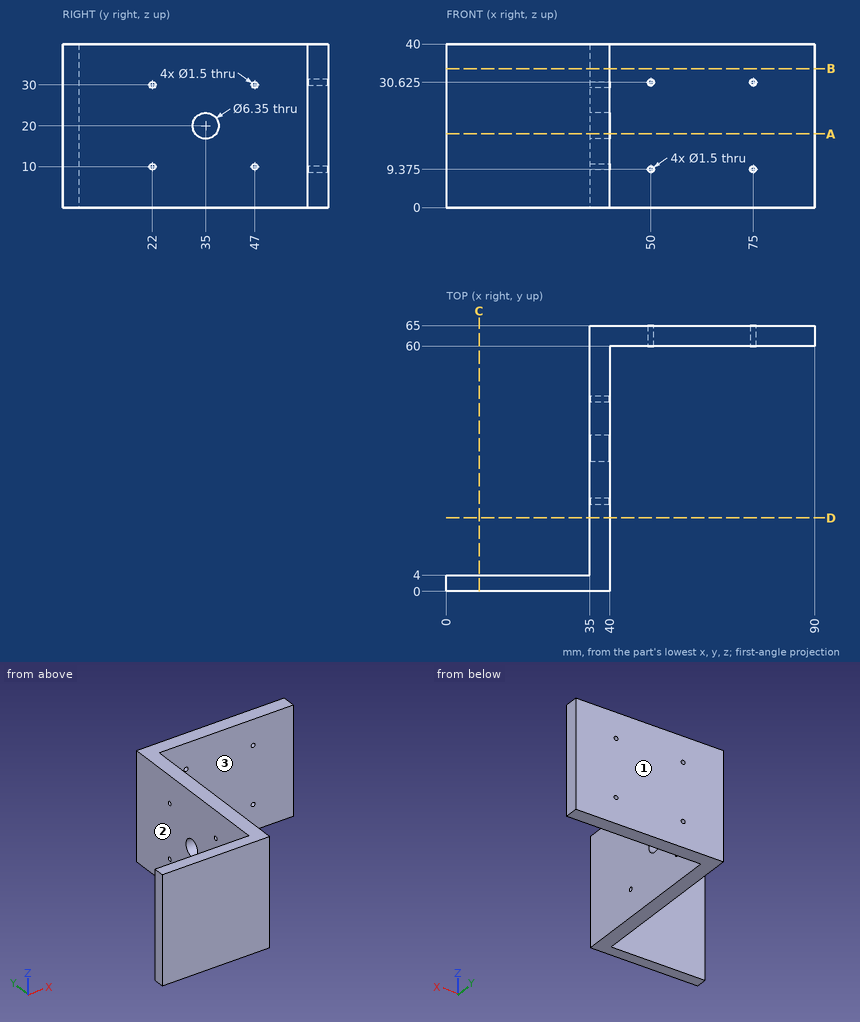
Geometry check sheet. Reference: drawing and pictorial views, mm from the part's lowest x, y, z. A direction names the side the tool comes from. Round coordinates to 2 decimals unless told otherwise and drop trailing zeros. Write each loop counter-clockwise with the first axis right and the second up, starting at its lowest first coordinate (ties: lowest second). Pieces come first, ordered by that corner, then holes.
Item 1: Section check A-A (z = 18). Record the boundary of the cut face in (x, y), plus the area to 3 significant figures.
Determined:
outline: (0, 0) - (40, 0) - (40, 32.53) - (35, 32.53) - (35, 4) - (0, 4) - close; (35, 37.47) - (40, 37.47) - (40, 60) - (90, 60) - (90, 65) - (35, 65) - close
area: 690 mm2
Item 2: Access from +Z, -Z, +X, -X, +Y, -Y to the whole of each face (thin tool, end or side, straight path). Record for the marked faces 1, 2 and 3.
Determined:
face 1: +Z, -Z, +X, -X, +Y
face 2: +Z, -Z, -X, +Y
face 3: +Z, -Z, +X, -Y
Item 3: Material ranges on line 1 along Y through (x, z) = (37, 30); line 2 along Z through (x, y) = (75, 61) (3 decimals); line 3 along Z through (x, y) = (36, 47), recorded low to high.
Determined:
line 1: y = 0 to 21.25, 22.75 to 46.25, 47.75 to 65
line 2: z = 0 to 8.625, 10.125 to 29.875, 31.375 to 40
line 3: z = 0 to 9.25, 10.75 to 29.25, 30.75 to 40
Item 4: Section check B-B (z = 34). Record the boundary of the cut face in (x, y).
Determined:
outline: (0, 0) - (40, 0) - (40, 60) - (90, 60) - (90, 65) - (35, 65) - (35, 4) - (0, 4) - close
Item 5: Go/stop test with flat-tipped pins: pin 1 Ø2 at (x, z) = (50, 30.625) entering from +Y; pin 2 Ø3 at (x, z) = (46, 32.5) entering from -Y; pin 3 Ø8 at (y, z) = (30.5, 34.5) entering from +X; pin 4 Ø17.5 at (x, z) = (15.5, 26) entering from +Y. Record where each tip stops, or that it passes through.
Determined:
pin 1: stops at y = 65
pin 2: stops at y = 60
pin 3: stops at x = 40
pin 4: stops at y = 4
Item 6: Section check C-C (x = 8). Record the boundary of the cut face in (y, z), plus the area to 3 significant figures.
Determined:
outline: (0, 0) - (4, 0) - (4, 40) - (0, 40) - close
area: 160 mm2
Item 7: Section check D-D (y = 18). Record the boundary of the cut face in (x, z).
Determined:
outline: (35, 0) - (40, 0) - (40, 40) - (35, 40) - close
